Input: dimensioned drawing with shaded views. Units: mm. Origin: part minimum x, y, z. Coordinates: 2 decimals unless noted, no trailing zeros. Order: outer loops, then holes, each group sorted by start corner. A loop starts at its lowest first (then second) coordinate and runs counter-clockwise, first axis right, second up. Notation, with made-up numbers: (35.5, 84.25) -> (48.5, 84.25) arc R22 cw to (48.5, 95.25) -> close; hole circle Ø4 at (-23, 42). An arc over 180 degrees is marked (long way). Answer as CSV lines item,"result".
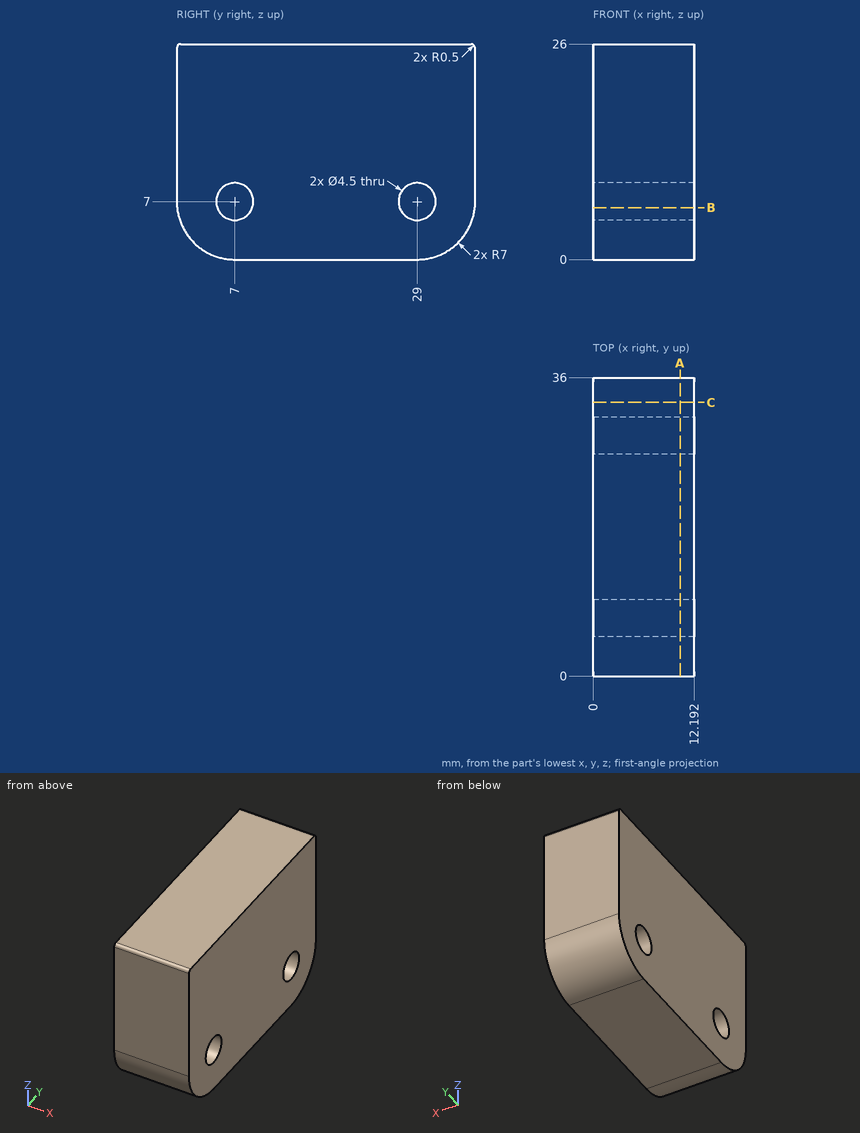
1. Cut plane C-C (y = 33). Return the cut outline in (x, z).
Findings:
outline,"(0, 1.26) -> (12.19, 1.26) -> (12.19, 26) -> (0, 26) -> close"
2. Cut plane A-A (x = 10.5). Return the cut outline in (y, z).
Findings:
outline,"(0, 7) arc R7 ccw to (7, 0) -> (29, 0) arc R7 ccw to (36, 7) -> (36, 25.5) arc R0.5 ccw to (35.5, 26) -> (0.5, 26) arc R0.5 ccw to (0, 25.5) -> close; hole circle Ø4.5 at (7, 7); hole circle Ø4.5 at (29, 7)"
3. Ray query, line 1 along Y through (x, z) = (6.5, 5); line 2 along Y through (x, z) = (5.75, 5.25); line 3 along Z through (x, y) = (6.25, 7). Return the intervals inside material, ascending.
Findings:
line 1,"y = 0.29 to 5.97, 8.03 to 27.97, 30.03 to 35.71"
line 2,"y = 0.22 to 5.59, 8.41 to 27.59, 30.41 to 35.78"
line 3,"z = 0 to 4.75, 9.25 to 26"
4. Cut plane B-B (z = 6.25). Return the cut outline in (x, y), plus the area to 3 significant figures.
Findings:
outline,"(0, 0.04) -> (12.19, 0.04) -> (12.19, 4.88) -> (0, 4.88) -> close; (0, 9.12) -> (12.19, 9.12) -> (12.19, 26.88) -> (0, 26.88) -> close; (0, 31.12) -> (12.19, 31.12) -> (12.19, 35.96) -> (0, 35.96) -> close"
area,"334 mm2"
